Study the drawing (mm; zero at the part's minimum x, y, z) and answer. A direction names the side the tool comes from. Coordinates: 2 decimals unless noted, no trailing zeros. Order: outer loops, then holes, each group sorted by start corner. A loop starts at its lowest first (then second) coordinate and runs counter-clockwise, first axis right, second up. Notation, with made-up numbers: (68, 44) -> (99, 44) arc R12 ccw to (99, 60) -> close; hole circle Ø5 at (0.25, 86.5). An arc over 180 degrees is marked (long way). Answer as CSV lines item,"result". Start each with the question number.
Item 1: Each of these flat-tipped pins is pushed along its axis until it touches: pin 1 Ø16 at (x, z) = (12.5, 8) entering from -Y; pin 2 Ø2 at (x, y) = (16.5, 15) entering from -Z; pin 3 Ø2 at (x, y) = (23.5, 18) entering from -Z. Where does it stop, or does it pass through?
Item 2: Section B-B (y = 12) is taken. Write down the section's boundary in (x, z), then the cut area to 3 significant figures.
Item 3: Which of the six approach directions +Z, -Z, +X, -X, +Y, -Y give full straight-line access (tool end or side, diameter ignored) to the marked faces 1, 2, 3, 4 and 5?
Item 4: Straight lines are drawn through the part: L1, parallel to X at y = 11.5, z = 23.5; L2, parallel to X at y = 26.25, z = 10; L3, parallel to Z at x = 22.75, y = 13.25. For each, find the intervals that lie inside material, in ascending order.
Item 5: Section C-C (z = 10) is taken. Write down the section's boundary in (x, y), then the cut area to 3 significant figures.
Item 6: Section A-A (x = 12.5) is taken. Write down the section's boundary in (y, z).
Item 7: Section D-D (y = 26) is taken. Write down the section's boundary in (x, z), then the cut area to 3 significant figures.
Item 8: For a pull along X with two mould halves and no side action, classify the marked faces 6, 7, 8 and 9 as pulls with the +X half, pulls with the -X half, needs draft (parallel to the pull), parting line crosses it, or undercut.
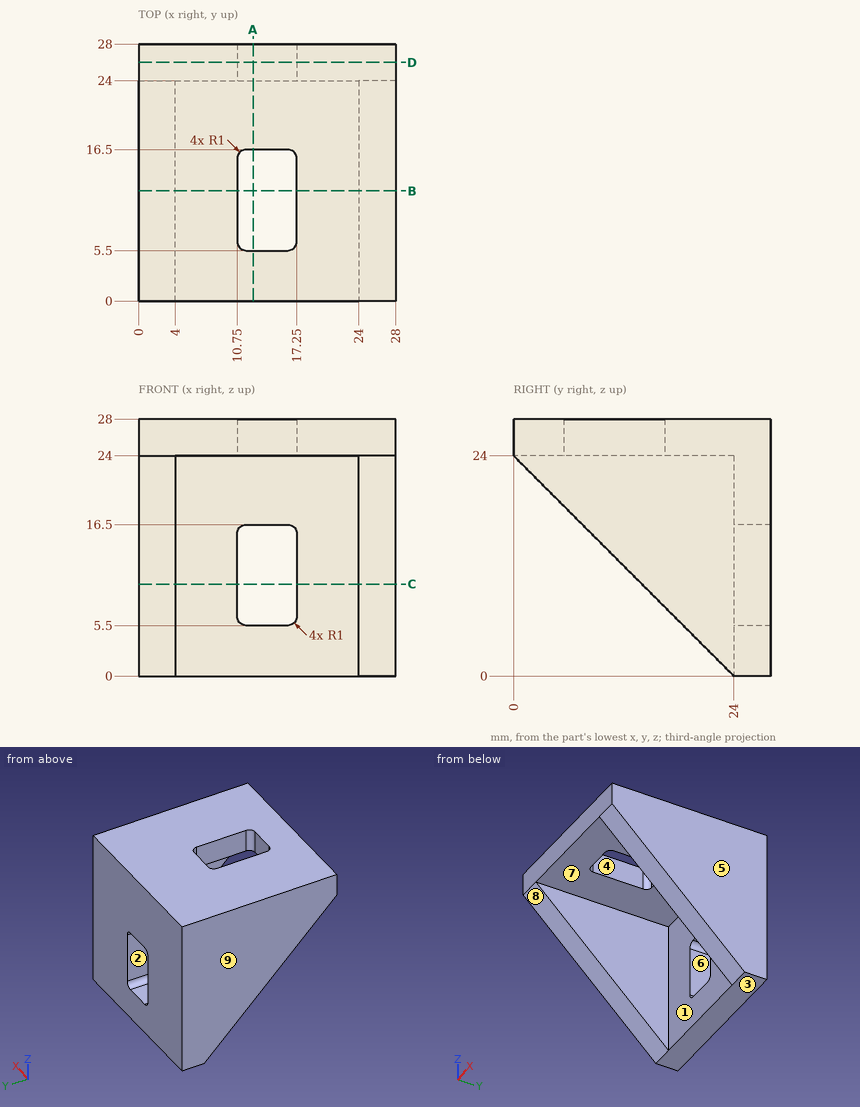
Checked values:
1,pin 1,"stops at y = 24"
1,pin 2,"stops at z = 24"
1,pin 3,"stops at z = 5.13"
2,outline,"(0, 12) -> (4, 12) -> (4, 24) -> (10.75, 24) -> (10.75, 28) -> (0, 28) -> close; (17.25, 24) -> (24, 24) -> (24, 12) -> (28, 12) -> (28, 28) -> (17.25, 28) -> close"
2,area,"182 mm^2"
3,face 1,"-Z, -Y"
3,face 2,"+Y, -Y"
3,face 3,"-Z, +X, -X, +Y, -Y"
3,face 4,"+Z, -Z"
3,face 5,"+Z, -Z, +X, +Y, -Y"
4,L1,"x = 0 to 4, 24 to 28"
4,L2,"x = 0 to 10.75, 17.25 to 28"
4,L3,"z = 24 to 28"
5,outline,"(0, 14) -> (4, 14) -> (4, 24) -> (10.75, 24) -> (10.75, 28) -> (0, 28) -> close; (17.25, 24) -> (24, 24) -> (24, 14) -> (28, 14) -> (28, 28) -> (17.25, 28) -> close"
5,area,"166 mm^2"
6,outline,"(0, 24) -> (5.5, 24) -> (5.5, 28) -> (0, 28) -> close; (16.5, 24) -> (24, 24) -> (24, 16.5) -> (28, 16.5) -> (28, 28) -> (16.5, 28) -> close; (24, 0) -> (28, 0) -> (28, 5.5) -> (24, 5.5) -> close"
7,outline,"(0, 0) -> (28, 0) -> (28, 28) -> (0, 28) -> close; hole (10.75, 6.5) arc R1 ccw to (11.75, 5.5) -> (16.25, 5.5) arc R1 ccw to (17.25, 6.5) -> (17.25, 15.5) arc R1 ccw to (16.25, 16.5) -> (11.75, 16.5) arc R1 ccw to (10.75, 15.5) -> close"
7,area,"713 mm^2"
8,face 6,"undercut"
8,face 7,"undercut"
8,face 8,"needs draft"
8,face 9,"pulls with the -X half"
